Solid Edge part; units mm, degrees
sketch "Sketch1" plane through (0, 0, 0) normal (0, -1, 0) x (1, 0, 0)
  line L0 (9.5, -11) -> (34.0656, -11)
  line L1 (34.0656, -11) -> (34.0656, -36)
  line L2 (-34.5, -36) -> (34.0656, -36)
  line L3 (-34.5, -11) -> (-34.5, -36)
  line L4 (-9.5, -11) -> (-34.5, -11)
  line L5 (-9.5, -10) -> (-9.5, -11)
  line L6 (-9.5, 0) -> (-9.5, -10)
  line L7 (-9.5, 0) -> (-19, 0)
  line L8 (-19, 0) -> (-19, 19)
  line L9 (-19, 19) -> (19, 19)
  line L10 (19, 0) -> (19, 19)
  line L11 (9.5, 0) -> (19, 0)
  line L12 (9.5, 0) -> (9.5, -10)
  line L13 (9.5, -10) -> (9.5, -11)
extrude "Protrusion1" add sketch "Sketch1" against normal blind 40
sketch "Sketch2" plane through (-0.2172, 20, -36) normal (0, 0, -1) x (1, 0, 0)
  circle A0 centre (-22.2078, 1.7938) radius 7.9323
extrude "ExtrudedProtrusion_2" add sketch "Sketch2" along normal blind 74.8424
sketch "Sketch3" plane through (-0.2172, 20, -36) normal (0, 0, -1) x (1, 0, 0)
  circle A0 centre (22.6421, 1.7938) radius 7.9323
extrude "ExtrudedProtrusion_3" add sketch "Sketch3" along normal blind 33.5499
sketch "Sketch4" plane through (14.2364, 0, 0) normal (1, 0, 0) x (0, 1, 0)
  circle A0 centre (6.0761, 0) radius 3.1934
  circle A1 centre (33.9239, 0) radius 3.1934
extrude "ExtrudedProtrusion_5" add sketch "Sketch4" along normal blind 2.6025
mirror "Mirror1" about plane through (0, 0, 0) normal (1, 0, 0) of "ExtrudedProtrusion_5"
The model under review builds one solid part; all positions refer to its coordinate system, in mm. A direction names the side the tool comes from. Give positions to 0.01 mm unless a question says otherwise; leave off trailing zeros. Write each loop counter-clockwise with the first axis right and the second up, starting at its lowest first coordinate (ties: lowest second). Pieces come first, ordered by that corner, then holes. Notation, with made-up numbers: (41.25, 34.25) -> (99.25, 34.25) arc R15 cw to (99.25, 57.25) -> close; hole circle Ø11 at (32.5, -29.5). An arc over 180 degrees is marked (long way). Answer in a Markdown table with one row per item.
1) Tool access review of faces 1 (the flat face through (22, 20, -11)), 2 (the cylindrical face through (-15.519, 33.854, -3.193)), 3 (the cylindrical face through (20.71, 10.46, -52.54)), 4 (the flat face through (23, 18, -69.55)), 5 (the flat face through (-14.236, 34, -1)): name each direction out of +Z, -Z, +X, -X, +Y, -Y from which nothing blocks a thin tool from reaching the whole face with its end or side.
Worked answers:
| item | result |
|---|---|
| face 1 | +X, +Y, -Y |
| face 2 | -X |
| face 3 | -Z |
| face 4 | -Z, +X, +Y, -Y |
| face 5 | +Y, -Y |
2) Add section C-C on z = 6.5. State the section outline as (x, y) points, plus the area to 3 significant figures.
Worked answers:
| item | result |
|---|---|
| outline | (-19, 0) -> (19, 0) -> (19, 40) -> (-19, 40) -> close |
| area | 1,520 mm² |
3) Add section A-A on x = 12.5. State the section outline as (y, z) points, plus the area to 3 significant figures.
Worked answers:
| item | result |
|---|---|
| outline | (0, -36) -> (40, -36) -> (40, -11) -> (0, -11) -> close; (0, 0) -> (40, 0) -> (40, 19) -> (0, 19) -> close |
| area | 1,760 mm² |
4) Mouldability with a two-part tool opening along X and no side actions: class faces 6 (the cylindrical face through (-15.519, 6.006, -3.193)), 7 (the cylindrical face through (-28.72, 13.38, -72.9)), 8 (the flat face through (-16.839, 34, -1)) as +X half, -X half, draft (parallel to the pull), parting line (faces both ways), or undercut.
Worked answers:
| item | result |
|---|---|
| face 6 | draft |
| face 7 | undercut |
| face 8 | -X half |
5) Clearance check with flat-ended pins moving along their axes: P1, Ø1.5, axis at x = -10.5, y = 17, coming from the -Z side; P2, Ø1, axis at y = 33.5, z = -2, coming from the +X side; P3, Ø8, axis at x = 25.5, y = 4.5, coming from the +Z side. State where each tip first meets the part, or that it passes through.
Worked answers:
| item | result |
|---|---|
| P1 | z = -36 |
| P2 | x = 16.84 |
| P3 | z = -11 |
6) For L1, parallel to Z at x = 12, y = 21; L2, parallel to Z at x = -24, y = 7.5; L3, parallel to Z at x = 0, y = 11, list the stretches that pass through material, from the lowest coordinate up. Write a range as [from, to].
Worked answers:
| item | result |
|---|---|
| L1 | [-36, -11], [0, 19] |
| L2 | [-36, -11] |
| L3 | [-36, 19] |
7) Add section D-D on y = 14. State the section outline as (x, z) points, plus the area to 3 significant figures.
Worked answers:
| item | result |
|---|---|
| outline | (-34.5, -36) -> (-29.15, -36) -> (-29.15, -110.84) -> (-15.7, -110.84) -> (-15.7, -36) -> (15.7, -36) -> (15.7, -69.55) -> (29.15, -69.55) -> (29.15, -36) -> (34.07, -36) -> (34.07, -11) -> (9.5, -11) -> (9.5, 0) -> (19, 0) -> (19, 19) -> (-19, 19) -> (-19, 0) -> (-9.5, 0) -> (-9.5, -11) -> (-34.5, -11) -> close |
| area | 4,100 mm² |
8) Add section B-B on x = 23.5. State the section outline as (y, z) points, plus the area to 3 significant figures.
Worked answers:
| item | result |
|---|---|
| outline | (0, -36) -> (10.35, -36) -> (10.35, -69.55) -> (26.07, -69.55) -> (26.07, -36) -> (40, -36) -> (40, -11) -> (0, -11) -> close |
| area | 1,530 mm² |
